Here's how the part is built. I have some questions about the finished solid (model axes, mm). A direction names the side the tool comes from. Round coordinates to 2 decimals unless told otherwise and drop trailing zeros. Write each loop counter-clockwise with the first axis right and the second up, starting at its lowest first coordinate (ties: lowest second). Pieces come first, ordered by that corner, then holes. Notation, with made-up numbers: (58, 27.5) - (107, 27.5) arc R7 ccw to (107, 32.5) - close; hole circle Ø7 at (32, 59). An arc over 180 degrees is marked (long way). One line per item, written item: value. Start each with the question number.
Item 1: For P1, Ø0.8, axis at y = 6, z = 9.5, coming from the +X side; P2, Ø5.5, axis at x = -11.5, y = 5.5, coming from the +Z side; P3, Ø1.2, axis at x = -97, z = 9, coming from the -Y side, each with a flat end and sliding along its axis, tell me the tip position at first contact or that it passes through.
Item 2: If I drill on line 1 (X direction, y = 13, z = 2.75); line 2 (Y direction, x = -89, z = 6); line 3 (Z direction, x = -12, y = 6.5), over which ranges is the centre line in solid material (lowest first)?
Item 3: Imagine slicing it at D-D, the plane z = 5.5. Please give me the cut outline in (x, y).
Item 4: Thinking about a two-plate mould opening in X: for faces 6 (the face through (-87.419, 8.883, 9.26)), 7 (the face through (-57, 0.769, 3)), 8 (the face through (0.001, 13.088, -0.566)), 9 (the face through (0.987, 15, 2)), which applies, released by +X, released by -X, zero draft, split by the parting line, or undercut?
Item 5: For faces 1 (the face through (-116.801, 15, 2)), 2 (the face through (-1.013, 16, 2)), 3 (the face through (-28, 0, 7)), 4 (the face through (-87.45, 3.52, 9.26)), 5 (the face through (-0.6, 3.3, 0)), which set-ups out of +Z, -Z, +X, -X, +Y, -Y let a thin tool reach every point of the face, with its end or its side?
Item 6: Imagine slicing it at A-A, the plane x = -95. Please give me the cut outline in (y, z).
Item 7: Imagine slicing it at B-B, the plane y = 24. Please give me the cut outline in (x, z).
Item 8: Imagine slicing it at C-C, the plane z = -5. Please give me the cut outline in (x, y).
```python
from build123d import *

# Parameters (mm, degrees)
F1_DEPTH  = 7
F2_R      = 7
F3_DEPTH  = 2
F4_R      = 7
F5_DEPTH  = 2
F6_W      = 32.3093086481
F6_H      = 2
F7_DEPTH  = 3
F8_W      = 32.3093086481
F8_H      = 1.5
F9_DEPTH  = 13
F11_W     = 10
F11_H     = 1.2
F12_DEPTH = 10
F13_DEPTH = 25
F14_R     = 3
F15_R     = 2
F16_R     = 1
F17_DEPTH = 117.7887811979
F18_R     = 3
F19_W     = 5.0336755812
F19_H     = 2.1570066456
F20_DEPTH = 2
F22_DEPTH = 2
F23_D     = 2.5


with BuildPart() as f1:
    # F0 (on Top) → F1 (new body)
    with BuildSketch(Plane.XY):
        Polygon((-114.8008331656, 27.8736967593), (-116.8008331656, 27.8736967593), (-116.8008331656, -1.2305311393), (0.9869479323, -1.2305311393), (0.9869479323, 27.8736967593), (-1.0130520677, 27.8736967593), (-1.0130520677, 0.7694688607), (-114.8008331656, 0.7694688607), align=None)
    extrude(amount=F1_DEPTH)

    # F2 (on face) → F3 (join)
    with BuildSketch(Plane(origin=(-116.8008331656, 0, 0), x_dir=(0, -1, 0), z_dir=(-1, 0, 0))):
        with Locations((-20.8736967593, 0)):
            Circle(F2_R)
    extrude(amount=-F3_DEPTH)

    # F4 (on face) → F5 (join)
    with BuildSketch(Plane(origin=(-1.0130520677, 0, 0), x_dir=(0, -1, 0), z_dir=(-1, 0, 0))):
        with Locations((-20.8736967593, 0)):
            Circle(F4_R)
    extrude(amount=-F5_DEPTH)

    # F6 (on face) → F7 (join)
    with BuildSketch(Plane.XY.offset(7)):
        with Locations((-97.5135117769, -0.2305311393)):
            Rectangle(F6_W, F6_H)
    extrude(amount=F7_DEPTH)

    # F8 (on face) → F9 (join)
    with BuildSketch(Plane(origin=(0, 0.7694688607, 0), x_dir=(-1, 0, 0), z_dir=(0, 1, 0))):
        with Locations((97.5135117769, 9.25)):
            Rectangle(F8_W, F8_H)
    extrude(amount=F9_DEPTH)

    # F11 (on face) → F12 (join)
    with BuildSketch(Plane.XZ.offset(1.2305311393)):
        with Locations((-13.2145643048, -0.6)):
            Rectangle(F11_W, F11_H)
    extrude(amount=-F12_DEPTH)

    # F10 (on face) → F13 (cut)
    with BuildSketch(Plane.XY.offset(10)):
        with BuildLine():
            ThreePointArc((-86.8486179709, 7.4843045808), (-87.4344044086, 8.8985181432), (-88.8486179709, 9.4843045808))
            Line((-88.8486179709, 9.4843045808), (-106.4697470069, 9.4843045808))
            ThreePointArc((-106.4697470069, 9.4843045808), (-107.8839605693, 8.8985181432), (-108.4697470069, 7.4843045808))
            Line((-108.4697470069, 7.4843045808), (-108.4697470069, 4.9521672986))
            ThreePointArc((-108.4697470069, 4.9521672986), (-108.4179393254, 4.4998989157), (-108.2652003167, 4.0710615092))
            ThreePointArc((-108.2652003167, 4.0710615092), (-107.9372939182, 3.5933788445), (-107.4862224218, 3.2297336335))
            ThreePointArc((-107.4862224218, 3.2297336335), (-106.996592653, 3.0228063513), (-106.4697470069, 2.9521672986))
            Line((-106.4697470069, 2.9521672986), (-88.8486179709, 2.9521672986))
            ThreePointArc((-88.8486179709, 2.9521672986), (-87.4344044086, 3.5379537363), (-86.8486179709, 4.9521672986))
            Line((-86.8486179709, 4.9521672986), (-86.8486179709, 7.4843045808))
        make_face()
    extrude(amount=-F13_DEPTH, mode=Mode.SUBTRACT)

    # F14
    f14_edges = [f1.edges().sort_by_distance(p)[0] for p in [
        (-113.668166, 13.769469, 9.25),
        (-81.358857, 13.769469, 9.25),
    ]]
    fillet(f14_edges, radius=F14_R)

    # F15
    f15_edges = [f1.edges().sort_by_distance(p)[0] for p in [
        (-97.513512, -1.230531, 10),
        (-97.513512, 0.769469, 8.5),
        (-13.214564, -1.230531, -1.2),
    ]]
    fillet(f15_edges, radius=F15_R)

    # F16
    f16_edges = [f1.edges().sort_by_distance(p)[0] for p in [
        (-13.214564, 0.769469, 0),
        (-1.013052, 0.769469, 3.25),
        (0.986948, -1.230531, 3.9),
        (-116.800833, -1.230531, 3.9),
        (-114.800833, 0.769469, 3.25),
        (-18.214564, 8.769469, -0.6),
        (-8.214564, 8.769469, -0.6),
        (-1.013052, 0.785409, 6.752009),
        (-114.800833, 0.785409, 6.752009),
        (-116.800833, -1.188344, 0.391381),
        (0.986948, -1.188344, 0.391381),
    ]]
    fillet(f16_edges, radius=F16_R)

    # F2 (on face) → F17 (cut, through all)
    with BuildSketch(Plane(origin=(-116.8008331656, 0, 0), x_dir=(0, -1, 0), z_dir=(-1, 0, 0))):
        with BuildLine():
            Line((-27.8736967593, 7), (-27.8736967593, 0))
            ThreePointArc((-27.8736967593, 0), (-25.8234442276, 4.9497474683), (-20.8736967593, 7))
            Line((-20.8736967593, 7), (-27.8736967593, 7))
        make_face()
    extrude(amount=-F17_DEPTH, mode=Mode.SUBTRACT)

    # F18
    f18_edges = [f1.edges().sort_by_distance(p)[0] for p in [
        (-115.800833, 13.873697, 0),
        (-0.013052, 13.873697, 0),
    ]]
    fillet(f18_edges, radius=F18_R)

    # F19 (on face) → F20 (join)
    with BuildSketch(Plane(origin=(-116.8008331656, 0, 0), x_dir=(0, -1, 0), z_dir=(-1, 0, 0))):
        with Locations((-28.0387327075, 0)):
            Rectangle(F19_W, F19_H)
    extrude(amount=-F20_DEPTH)

    # F21 (on face) → F22 (join)
    with BuildSketch(Plane(origin=(-1.0130520677, 0, 0), x_dir=(0, -1, 0), z_dir=(-1, 0, 0))):
        with BuildLine():
            Line((-27.7901142267, 1.0785033228), (-30.5555704981, 1.0785033228))
            Line((-30.5555704981, 1.0785033228), (-30.5555704981, -1.0785033228))
            Line((-30.5555704981, -1.0785033228), (-27.7901142267, -1.0785033228))
            ThreePointArc((-27.7901142267, -1.0785033228), (-27.8736967593, 0), (-27.7901142267, 1.0785033228))
        make_face()
    extrude(amount=-F22_DEPTH)

    # F23 (through all)
    with Locations(Plane(origin=(-116.8008331656, 0, 0), x_dir=(0, -1, 0), z_dir=(-1, 0, 0))):
        with Locations((-20.8736967593, 0)):
            Hole(F23_D / 2)


solid = f1.part
```
Values follow:
1. P1: stops at x = -81.36
1. P2: stops at z = 0
1. P3: stops at y = -1.19
2. line 1: x = -116.8 to -114.8, -1.01 to 0.99
2. line 2: y = -1.23 to 0.77
2. line 3: z = -1.2 to 0
3. outline: (-116.8, -0.23) arc R1 ccw to (-115.8, -1.23) - (-0.01, -1.23) arc R1 ccw to (0.99, -0.23) - (0.99, 25.2) - (-1.01, 25.2) - (-1.01, 1.77) arc R1 cw to (-2.01, 0.77) - (-113.8, 0.77) arc R1 cw to (-114.8, 1.77) - (-114.8, 25.2) - (-116.8, 25.2) - close
4. face 6: undercut
4. face 7: undercut
4. face 8: zero draft
4. face 9: released by +X
5. face 1: +Z, -Z, -X, +Y, -Y
5. face 2: +Z, -Z, +Y
5. face 3: +Z, +X, +Y, -Y
5. face 4: +Z, -Z
5. face 5: -Z, +X, -Y
6. outline: (-1.23, 0.8) arc R2 ccw to (-1.06, 0) - (0.77, 0) - (0.77, 6.5) arc R2 cw to (2.77, 8.5) - (2.95, 8.5) - (2.95, 10) - (0.77, 10) arc R2 ccw to (-1.23, 8) - close; (9.48, 8.5) - (13.77, 8.5) - (13.77, 10) - (9.48, 10) - close
7. outline: (-116.8, -6.26) - (-114.8, -6.26) - (-114.8, 6.26) - (-116.8, 6.26) - close; (-1.01, -6.26) - (0.99, -6.26) - (0.99, 6.26) - (-1.01, 6.26) - close
8. outline: (-116.8, 15.97) - (-114.8, 15.97) - (-114.8, 25.77) - (-116.8, 25.77) - close; (-1.01, 15.97) - (0.99, 15.97) - (0.99, 25.77) - (-1.01, 25.77) - close
